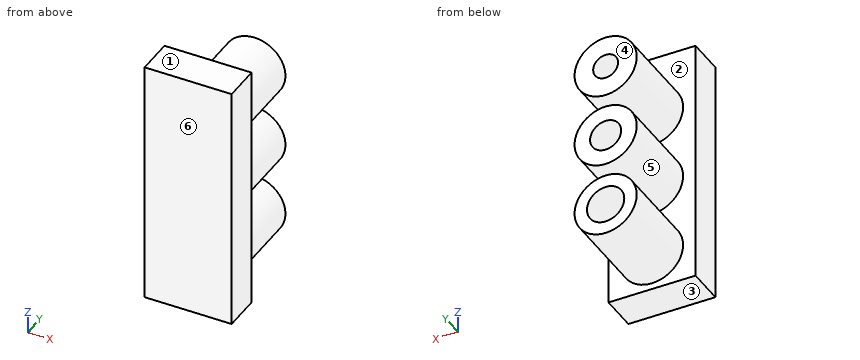
Autodesk Inventor part; units mm, degrees
ref_plane "YZ Plane" through (0, 0, 0) normal (1, 0, 0) x (0, 1, 0)
ref_plane "XZ Plane" through (0, 0, 0) normal (0, 1, 0) x (-1, 0, 0)
ref_plane "XY Plane" through (0, 0, 0) normal (0, 0, 1) x (1, 0, 0)
sketch "Sketch1" plane through (0, 0, 0) normal (0, 1, 0) x (-1, 0, 0)
  line L0 (0, 0) -> (7, 0)
  line L1 (7, 0) -> (7, -20)
  line L2 (7, -20) -> (0, -20)
  line L3 (0, -20) -> (0, 0)
  line L4 (0, 0) -> (0, -5)
  line L5 (0, -5) -> (3.5, -5)
  circle A0 centre (3.5, -5) radius 2.5
  circle A1 centre (3.5, -5) radius 1
  line L6 (0, -5) -> (0, -11)
  line L7 (0, -11) -> (3.5, -11)
  circle A2 centre (3.5, -11) radius 2.5
  circle A3 centre (3.5, -11) radius 1.25
  line L8 (0, -11) -> (0, -17)
  line L9 (0, -17) -> (3.5, -17)
  circle A4 centre (3.5, -17) radius 2.5
  circle A5 centre (3.5, -17) radius 1.5
  dimension "d0" = 7
  dimension "d1" = 20
  dimension "d2" = 5
  dimension "d3" = 3.5
  dimension "d4" = 5
  dimension "d5" = 2
  dimension "d6" = 6
  dimension "d7" = 3.5
  dimension "d8" = 5
  dimension "d9" = 2.5
  dimension "d10" = 6
  dimension "d11" = 3.5
  dimension "d12" = 5
  dimension "d13" = 3
extrude "Extrusion1" add sketch "Sketch1" along normal blind 3 contours L0 L1 L2 L3
extrude "Extrusion2" add sketch "Sketch1" along normal blind 3 contours A1 | A3 | A5
extrude "Extrusion3" add sketch "Sketch1" along normal blind 10 contours A0 | A2 | A4
properties part number "HoleSizeTest"
Could you check a few things on this model? Use its own coordinates, in mm. Face numbers are marked on the shaded views. A direction names the side the tool comes from. Round coordinates to 2 decimals unless told otherwise and drop trailing zeros. Loops run counter-clockwise (first coordinate to the right, second up) from the corner with the lowest first, then second, coordinate; pieces in that order, holes last. Notation, with made-up numbers: (1.25, 49.5) -> (39.25, 49.5) arc R25 ccw to (39.25, 79.5) -> close; hole circle Ø10 at (-3.75, 43.5). An arc over 180 degrees is marked (long way). Put each result on its own line as item: value.
Q1. I want a section at B-B on x = -3.5. Write out the boundary of the cut face in (y, z).
Checks:
outline: (0, -20) -> (3, -20) -> (3, -19.5) -> (10, -19.5) -> (10, -18.5) -> (3, -18.5) -> (3, -15.5) -> (10, -15.5) -> (10, -14.5) -> (3, -14.5) -> (3, -13.5) -> (10, -13.5) -> (10, -12.25) -> (3, -12.25) -> (3, -9.75) -> (10, -9.75) -> (10, -8.5) -> (3, -8.5) -> (3, -7.5) -> (10, -7.5) -> (10, -6) -> (3, -6) -> (3, -4) -> (10, -4) -> (10, -2.5) -> (3, -2.5) -> (3, 0) -> (0, 0) -> close
Q2. For pin 1 Ø2 at (y, z) = (5.5, -6.5) entering from -X; pin 2 Ø1.5 at (x, y) = (-5.5, 8) entering from -Z; pin 3 Ø2 at (x, y) = (-5.5, 7.5) entering from -Z, each with a flat end and sliding along its axis, tell me the tip position at first contact or that it passes through.
Checks:
pin 1: x = -5.95
pin 2: z = -19.17
pin 3: z = -19.29
Q3. Please list where these lines run through material, in increasing order: line 1 (Z direction, x = -3.5, y = 6); line 2 (X direction, y = 5.75, z = -5); line 3 (X direction, y = 8.5, z = -17). Write a range as from..to.
Checks:
line 1: -19.5..-18.5, -15.5..-14.5, -13.5..-12.25, -9.75..-8.5, -7.5..-6, -4..-2.5
line 2: -6..-4.5, -2.5..-1
line 3: -6..-5, -2..-1
Q4. I want a section at C-C on z = -11. Write out the boundary of the cut face in (x, y).
Checks:
outline: (-7, 0) -> (0, 0) -> (0, 3) -> (-1, 3) -> (-1, 10) -> (-2.25, 10) -> (-2.25, 3) -> (-4.75, 3) -> (-4.75, 10) -> (-6, 10) -> (-6, 3) -> (-7, 3) -> close
Q5. I want a section at A-A on y = 5.5. Write out the boundary of the cut face in (x, z).
Checks:
outline: circle Ø5 at (-3.5, -17); circle Ø5 at (-3.5, -11); circle Ø5 at (-3.5, -5); hole circle Ø3 at (-3.5, -17); hole circle Ø2.5 at (-3.5, -11); hole circle Ø2 at (-3.5, -5)
Q6. Thinking about a two-plate mould opening in Z: for the marked faces 1, 2, 3 and 4, which applies, pulls with the +Z half, pulls with the -Z half, needs draft (parallel to the pull), parting line crosses it, or undercut?
Checks:
face 1: pulls with the +Z half
face 2: undercut
face 3: pulls with the -Z half
face 4: needs draft
Q7. I want a section at D-D on x = -5.5. Write out the boundary of the cut face in (y, z).
Checks:
outline: (0, -20) -> (3, -20) -> (3, -18.5) -> (10, -18.5) -> (10, -15.5) -> (3, -15.5) -> (3, -12.5) -> (10, -12.5) -> (10, -9.5) -> (3, -9.5) -> (3, -6.5) -> (10, -6.5) -> (10, -3.5) -> (3, -3.5) -> (3, 0) -> (0, 0) -> close
Q8. Which directions (+Z, -Z, +X, -X, +Y, -Y) give clear straight access to the entire face, cutting with the end or side of a thin tool? Please do the marked faces 5 and 6.
Checks:
face 5: +Y
face 6: +Z, -Z, +X, -X, -Y
